Autodesk Inventor part; units mm, degrees
ref_plane "YZ Plane" through (0, 0, 0) normal (1, 0, 0) x (0, 1, 0)
ref_plane "XZ Plane" through (0, 0, 0) normal (0, 1, 0) x (-1, 0, 0)
ref_plane "XY Plane" through (0, 0, 0) normal (0, 0, 1) x (1, 0, 0)
sketch "Sketch1" plane through (0, 0, 0) normal (0, 0, 1) x (1, 0, 0)
  line L0 (0, 0) -> (50.8, 0)
  line L1 (50.8, 0) -> (50.8, 25.4)
  line L2 (50.8, 25.4) -> (0, 25.4)
  line L3 (0, 25.4) -> (0, 0)
  line L4 (1.5875, 1.5875) -> (49.2125, 1.5875)
  line L5 (49.2125, 1.5875) -> (49.2125, 23.8125)
  line L6 (49.2125, 23.8125) -> (1.5875, 23.8125)
  line L7 (1.5875, 23.8125) -> (1.5875, 1.5875)
  dimension "d0" = 50.8
  dimension "d1" = 25.4
  dimension "d2" = 1.5875
extrude "Extrusion1" add sketch "Sketch1" along normal blind 601.9292
sketch "Sketch2" plane through (0, 25.4, 0) normal (0, 1, 0) x (1, 0, 0)
  line L0 (125.8687, -681.3224) -> (26.7439, -601.9292)
  line L1 (26.7439, -601.9292) -> (85.6181, -528.4229)
  line L2 (85.6181, -528.4229) -> (184.7429, -607.8161)
  line L3 (184.7429, -607.8161) -> (125.8687, -681.3224)
  line L4 (-52.6493, -701.054) -> (26.7439, -601.9292)
  line L5 (26.7439, -601.9292) -> (-41.6165, -547.1765)
  line L6 (-41.6165, -547.1765) -> (-121.0097, -646.3013)
  line L7 (-121.0097, -646.3013) -> (-52.6493, -701.054)
  line L8 (50.8, 0) -> (0, 0)
  line L9 (0, 0) -> (0, -601.9292)
  line L10 (50.8, -601.9292) -> (0, -601.9292)
  line L11 (50.8, 0) -> (50.8, -601.9292)
  line L12 (0, 0) -> (0, -601.9292)
  point P0 (50.8, -571.8944)
  point P1 (0, -580.5089)
  dimension "d6" = 127
  dimension "d7" = 127
  dimension "d9" = 38.481
  dimension "d16" = 34.2646
extrude "Extrusion2" cut sketch "Sketch2" against normal blind 25.4 contours L0 L10 L11 L1 L2 L3 | L10 L9 L5 | L1 L11 L10 | L4 L7 L6 L5 L9 L10
sketch "Sketch3" plane through (0, 25.4, 0) normal (0, 1, 0) x (1, 0, 0)
  line L0 (0, 0) -> (59.8042, 74.6674)
  line L1 (59.8042, 74.6674) -> (161.4042, -6.7083)
  line L2 (161.4042, -6.7083) -> (101.6, -81.3757)
  line L3 (101.6, -81.3757) -> (0, 0)
  line L4 (50.8, 0) -> (0, 0)
  line L5 (50.8, 0) -> (50.8, -571.8944)
  line L6 (0, -580.5089) -> (26.7439, -601.9292)
  point P0 (50.8, -40.6878)
extrude "Extrusion3" cut sketch "Sketch3" against normal blind 25.4 contours L4 L5 L3
sketch "Sketch4" plane through (0, 25.4, 580.5089) normal (0, 1, 0) x (1, 0, 0)
  line L0 (-37.1172, 580.5089) -> (145.2482, 580.5089) construction
  line L1 (0, 580.5089) -> (0, 0) construction
  point P0 (25.4, 217.3651)
  point P1 (25.4, 24.1981)
  point P2 (26.7439, -21.4203)
  dimension "d17" = 25.4
  dimension "d20" = 25.4
  dimension "d28" = 238.7854
  dimension "d29" = 45.6184
hole "Hole1" at (25.4, 25.4, 363.1438) at (25.4, 25.4, 556.3108) direction (0, -1, 0) diameter 28.575 depth 25.4 tip angle 118
ref_plane "Work Plane1" through (25.4, 0, 571.8944) normal (1, 0, 0) x (0, 0, -1)
properties part number "SUP_010_4BarBar" material "Aluminum 6061"
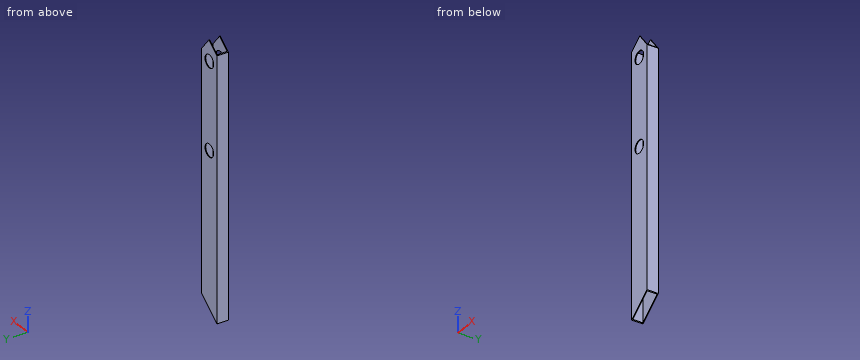
The model under review builds one solid part; all positions refer to its coordinate system, in mm. Give positions to 0.01 mm unless a question says otherwise; leave off trailing zeros. Order: outer loops, then holes, each group sorted by start corner. A loop starts at its lowest first (then second) coordinate and runs counter-clockwise, first axis right, second up. Notation, with made-up numbers: (89.5, 79.5) - (109.5, 79.5) arc R12 cw to (109.5, 87.5) - close; hole circle Ø7 at (32, 8.25). An arc over 180 degrees is marked (long way). Use CSV: the item, a comma, the result in double quotes. Start each with the question number.
Q1. Clearance check with a flat-ended pin moving along its axis: pin 1 Ø5 at (x, z) = (36.5, 404.5) entering from -Y. State where the tip first meets the part, or that it passes through.
Q2. We need section A-A, the plane z = 299. Write out the cut boundary in (x, y), and give its area (3 significant figures).
Q3. We need section B-B, the plane y = 6. Write out the cut boundary in (x, z), and give its area (3 significant figures).
Q4. We need section C-C, the plane x = 34.5. Write out the cut boundary in (y, z).
Q5. To check wall thickness, follow line 1 along X through (y, z) = (19.25, 309); line 2 along Y through (x, z) = (4, 280); line 3 along Z through (x, y) = (26.5, 24.25). State the ranges of each line that lie inside material, in increasing order. Write a range as [from, to].
Outcome:
1,pin 1,"stops at y = 0"
2,outline,"(0, 0) - (50.8, 0) - (50.8, 25.4) - (0, 25.4) - close; hole (1.59, 1.59) - (49.21, 1.59) - (49.21, 23.81) - (1.59, 23.81) - close"
2,area,"232 mm^2"
3,outline,"(0, 0) - (1.59, 1.27) - (1.59, 581.78) - (0, 580.51) - close; (49.21, 39.42) - (50.8, 40.69) - (50.8, 571.89) - (49.21, 573.88) - close"
3,area,"1,770 mm^2"
4,outline,"(0, 27.63) - (1.59, 27.63) - (1.59, 352.13) - (0, 352.13) - close; (0, 374.16) - (1.59, 374.16) - (1.59, 545.3) - (0, 545.3) - close; (0, 567.33) - (1.59, 567.33) - (1.59, 592.25) - (0, 592.25) - close; (23.81, 27.63) - (25.4, 27.63) - (25.4, 352.13) - (23.81, 352.13) - close; (23.81, 374.16) - (25.4, 374.16) - (25.4, 545.3) - (23.81, 545.3) - close; (23.81, 567.33) - (25.4, 567.33) - (25.4, 592.25) - (23.81, 592.25) - close"
5,line 1,"x = [0, 1.59], [49.21, 50.8]"
5,line 2,"y = [0, 1.59], [23.81, 25.4]"
5,line 3,"z = [21.22, 348.9], [377.39, 542.07], [570.56, 601.73]"
